The listing builds one solid part. Answer for the finished solid, in the listing's coordinates (mm). A direction names the side the tool comes from. Round coordinates to 2 decimals unless told otherwise and drop trailing zeros. Order: outer loops, then holes, each group sorted by start corner. A loop starts at its lowest first (then second) coordinate and runs counter-clockwise, first axis right, second up. Notation, with made-up numbers: (85, 77.5) - (127, 77.5) arc R7 ccw to (127, 84.5) - close; hole circle Ø7 at (38, 20.25). An arc over 180 degrees is marked (long way). Write item = value, one per line.
from build123d import *

# Parameters (mm, degrees)
SKETCH1_W            = 34
SKETCH1_H            = 55
BOSS_EXTRUDE1_DEPTH  = 3
SKETCH2_R            = 1.5
CUT_EXTRUDE1_DEPTH   = 3
CUT_EXTRUDE4_DEPTH   = 3
LPATTERN1_COUNT      = 2
LPATTERN1_PITCH      = 25.5
SKETCH5_W            = 6
SKETCH5_H            = 3
CUT_EXTRUDE5_DEPTH   = 3
LPATTERN2_COUNT      = 3
LPATTERN2_PITCH      = 10
LPATTERN2_COUNT_DIR2 = 2
LPATTERN2_PITCH_DIR2 = 35
SKETCH6_R            = 4.5
CUT_EXTRUDE6_DEPTH   = 3
CUT_EXTRUDE7_DEPTH   = 3
FILLET9_R            = 3
FILLET10_R           = 3


with BuildPart() as part:
    # Sketch1 → Boss-Extrude1 (new body)
    with BuildSketch(Plane(origin=(0, 0, 0), x_dir=(1, 0, 0), z_dir=(0, 1, 0))):
        Rectangle(SKETCH1_W, SKETCH1_H)
    extrude(amount=BOSS_EXTRUDE1_DEPTH)

    # Sketch2 → Cut-Extrude1 (cut)
    with BuildSketch(Plane(origin=(0, 3, 0), x_dir=(1, 0, 0), z_dir=(0, 1, 0))):
        with Locations(Location((-3, 2.680652708, 0), (0, 0, 270))):
            Circle(SKETCH2_R)
    extrude(amount=-CUT_EXTRUDE1_DEPTH, mode=Mode.SUBTRACT)

    # Sketch4 → Cut-Extrude4 (cut)
    with BuildSketch(Plane(origin=(0, 3, 0), x_dir=(1, 0, 0), z_dir=(0, 1, 0))):
        Polygon((-13.55, -16.7), (-11.95, -16.7), (-11.95, -18.3), (-10.35, -18.3), (-10.35, -19.9), (-11.95, -19.9), (-11.95, -21.5), (-13.55, -21.5), (-13.55, -19.9), (-15.15, -19.9), (-15.15, -18.3), (-13.55, -18.3), align=None)
    cut_extrude4 = extrude(amount=-CUT_EXTRUDE4_DEPTH, mode=Mode.SUBTRACT)

    # LPattern1: Cut-Extrude4 ×2
    with Locations(*[(i * LPATTERN1_PITCH, 0, 0) for i in range(1, LPATTERN1_COUNT)]):
        add(cut_extrude4, mode=Mode.SUBTRACT)

    # Sketch5 → Cut-Extrude5 (cut)
    with BuildSketch(Plane(origin=(0, 3, 0), x_dir=(1, 0, 0), z_dir=(0, 1, 0))):
        with Locations((-10, 23)):
            Rectangle(SKETCH5_W, SKETCH5_H)
    cut_extrude5 = extrude(amount=-CUT_EXTRUDE5_DEPTH, mode=Mode.SUBTRACT)

    # LPattern2: Cut-Extrude5 3 × 2
    with Locations(*[(i * LPATTERN2_PITCH, 0, j * LPATTERN2_PITCH_DIR2) for i in range(LPATTERN2_COUNT) for j in range(LPATTERN2_COUNT_DIR2) if (i, j) != (0, 0)]):
        add(cut_extrude5, mode=Mode.SUBTRACT)

    # Sketch6 → Cut-Extrude6 (cut)
    with BuildSketch(Plane(origin=(0, 3, 0), x_dir=(1, 0, 0), z_dir=(0, 1, 0))):
        with Locations(Location((0, 15, 0), (0, 0, 270))):
            Circle(SKETCH6_R)
    extrude(amount=-CUT_EXTRUDE6_DEPTH, mode=Mode.SUBTRACT)

    # Sketch8 → Cut-Extrude7 (cut)
    with BuildSketch(Plane(origin=(0, 3, 0), x_dir=(1, 0, 0), z_dir=(0, 1, 0))):
        Polygon((0.853324812, 11.496881851), (-2.905445672, 12.864962424), (-4.615546388, 8.16649932), (-0.856775905, 6.798418747), align=None)
    extrude(amount=-CUT_EXTRUDE7_DEPTH, mode=Mode.SUBTRACT)

    # Fillet9
    fillet9_edges = [part.edges().sort_by_distance(p)[0] for p in [
        (-3.258112517, 1.5, -11.89601823),
    ]]
    fillet(fillet9_edges, radius=FILLET9_R)

    # Fillet10
    fillet10_edges = [part.edges().sort_by_distance(p)[0] for p in [
        (0.500657966, 1.5, -10.527937657),
    ]]
    fillet(fillet10_edges, radius=FILLET10_R)


solid = part.part
Q1. Section B-B on z = -15 is taken. Determine the outline of the cut face in (x, y).
Model answer:
outline = (-17, 0) - (-4.5, 0) - (-4.5, 3) - (-17, 3) - close; (4.5, 0) - (17, 0) - (17, 3) - (4.5, 3) - close
Q2. Section D-D on y = 0.5 is taken. Count the separate pieces of the cut face and the enclosed holes in it, then the cut area to 3 significant figures.
Model answer:
separate_pieces = 1
enclosed_holes = 10
area = 1,650 mm^2
Q3. Find the intervals of material crossed by line 1 (Z direction, x = 12, y = 1); line 2 (X direction, y = 0.2, z = 13); line 3 (Z direction, x = 9, y = 1.2), in increasing order. Write a range as from..to.
Model answer:
line_1 = -27.5..-24.5, -21.5..10.5, 13.5..16.7, 21.5..27.5
line_2 = -17..-13, -7..-3, 3..7, 13..17
line_3 = -27.5..-24.5, -21.5..10.5, 13.5..27.5
Q4. Section A-A on z = 19 is taken. Determine the outline of the cut face in (x, y), then the cut area to 3 significant figures.
Model answer:
outline = (-17, 0) - (-15.15, 0) - (-15.15, 3) - (-17, 3) - close; (-10.35, 0) - (10.35, 0) - (10.35, 3) - (-10.35, 3) - close; (15.15, 0) - (17, 0) - (17, 3) - (15.15, 3) - close
area = 73.2 mm^2
Q5. Determine the mould class of faces 3 (the face through (13, 2, -23)), 4 (the face through (-7, 2, 12)), 5 (the face through (0, 0, 0)) for opening direction Z: released by +Z, released by -Z, zero draft, split by the parting line, or undercut.
Model answer:
face_3 = undercut
face_4 = undercut
face_5 = zero draft
Q6. For faces 1 (the face through (17, 1, 0)), 2 (the face through (-11.95, 2, 21)), determine the directions among +Z, -Z, +X, -X, +Y, -Y from which every point of the face is accessible in a straight line to the end or side of a thin tool.
Model answer:
face_1 = +Z, -Z, +X, +Y, -Y
face_2 = +Y, -Y
Q7. Section C-C on x = -9.5 is taken. Determine the outline of the cut face in (y, z).
Model answer:
outline = (0, -27.5) - (3, -27.5) - (3, -24.5) - (0, -24.5) - close; (0, -21.5) - (3, -21.5) - (3, 10.5) - (0, 10.5) - close; (0, 13.5) - (3, 13.5) - (3, 27.5) - (0, 27.5) - close
